Design review of the part built by this model. Coordinates are the model's own, in mm. Face numbers are marked on the shaded views. A direction names the side the tool comes from. Coordinates: 2 decimals unless noted, no trailing zeros. Loops run counter-clockwise (first coordinate to the right, second up) from the corner with the lowest first, then second, coordinate; pieces in that order, holes last. Notation, with made-up numbers: (39, 65.5) - (96, 65.5) arc R20 cw to (96, 83.5) - close; hole circle Ø4 at (31, -30). An arc over 180 degrees is marked (long way). Answer in a Markdown table with one row per item. Add a question column.
(1) We need section C-C, the plane y = -8.75. Write out the cut boundary in (x, z), plus the area to 3 significant figures.
(2) We need section D-D, the plane x = 28. Write out the cut boundary in (y, z), plus the area to 3 significant figures.
(3) We need section A-A, the plane y = -3.75. Write out the cut boundary in (x, z), plus the area to 3 significant figures.
(4) For the marked faces 1, 2 and 3, list the 3-axis set-ups (+Z, -Z, +X, -X, +Y, -Y) from which the entire face can be reached by the end or side of a thin tool; tool diameter is ignored.
(5) To check wall thickness, follow L1, parallel to X at y = -2.4, z = -89.63; L2, parallel to X at y = -7.8, z = -89.63; L3, parallel to Y at x = 27.5, z = -9. State the ranges of each line that lie inside material, in increasing order. Write a range as [from, to].
(6) We need section B-B, the plane z = -59.63. Write out the cut boundary in (x, y).
(7) Clearance check with flat-ended pins moving along their axes: pin 1 (2 mm diameter, centred on x = 28, y = -7, fed in from -Z); pin 2 (0.6 mm diameter, centred on x = 7, y = -10, fed in from -Z); pin 3 (7.5 mm diameter, centred on x = 5, z = -89.63, fed in from -Y); pin 4 (1.3 mm diameter, centred on x = 5.5, z = -39.5, fed in from -Y). State where each tip first meets the part, or that it passes through.
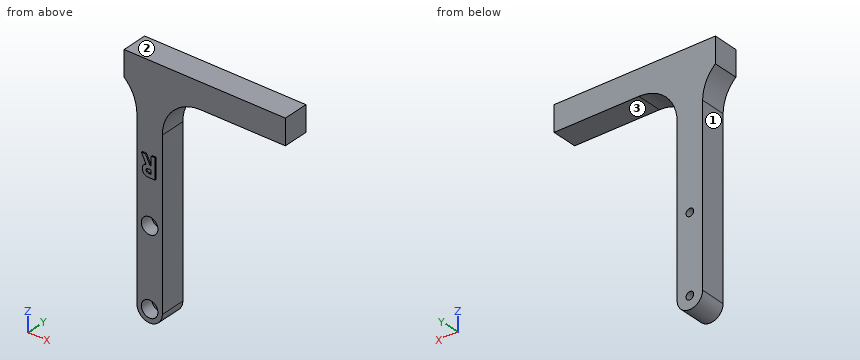
from build123d import *

# Parameters (mm, degrees)
BOSS_EXTRUDE1_DEPTH = 10
SKETCH2_R           = 1.5
CUT_EXTRUDE1_DEPTH  = 112.585820336
BOSS_EXTRUDE2_DEPTH = 0.5
SKETCH5_R           = 3.25
CUT_EXTRUDE2_DEPTH  = 5
FILLET1_R           = 15


with BuildPart() as part:
    # Sketch1 → Boss-Extrude1 (new body)
    with BuildSketch(Plane(origin=(0, 0, 0), x_dir=(1, 0, 0), z_dir=(0, 1, 0))):
        with BuildLine():
            Line((0, 0), (10, 0))
            Line((10, 0), (58.28, 0))
            Line((58.28, 0), (58.28, 10))
            Line((58.28, 10), (10, 10))
            Line((10, 10), (10, 89.63))
            ThreePointArc((10, 89.63), (5, 94.63), (0, 89.63))
            Line((0, 89.63), (0, 10))
            Line((0, 10), (-5, 10))
            Line((-5, 10), (-5, 0))
            Line((-5, 0), (0, 0))
        make_face()
    extrude(amount=BOSS_EXTRUDE1_DEPTH)

    # Sketch2 → Cut-Extrude1 (cut, through all)
    with BuildSketch(Plane(origin=(0, 10, 0), x_dir=(1, 0, 0), z_dir=(0, 1, 0))):
        with Locations(Location((5, 89.63, 0), (0, 0, 270))):
            Circle(SKETCH2_R)
        with Locations(Location((5, 59.63, 0), (0, 0, 270))):
            Circle(SKETCH2_R)
    extrude(amount=-CUT_EXTRUDE1_DEPTH, mode=Mode.SUBTRACT)

    # Sketch4 → Boss-Extrude2 (add)
    with BuildSketch(Plane(origin=(0, 10, 0), x_dir=(1, 0, 0), z_dir=(0, 1, 0))):
        with BuildLine():
            Line((7.461538462, 41.930004151), (5.788461538, 41.930004151))
            add(Edge.make_bspline(
                [(5.788461538, 41.930004151), (5.677871663, 41.92961162), (5.465176181, 41.928856674), (5.158480914, 41.916945611), (4.876739133, 41.900370391), (4.619533695, 41.875076164), (4.386974636, 41.841539077), (4.178828878, 41.802004401), (3.995102505, 41.756946162), (3.834246039, 41.700800041), (3.689081032, 41.637468067), (3.553767063, 41.564698468), (3.425318906, 41.483301557), (3.304595098, 41.391135559), (3.19054652, 41.289858519), (3.082958012, 41.179368492), (2.983349901, 41.058728567), (2.892338963, 40.928701036), (2.809389819, 40.791915054), (2.736080173, 40.648182815), (2.676464647, 40.497404362), (2.62378794, 40.341758769), (2.585846614, 40.179021052), (2.559458976, 40.010775491), (2.540138981, 39.836429843), (2.539028173, 39.71798715), (2.538461538, 39.657568254)],
                knots=[0, 0, 0, 0, 1.749336639, 3.364467119, 4.854658419, 6.213483162, 7.451590619, 8.570285859, 9.5643256, 10.440900261, 11.26203566, 12.067320669, 12.869050712, 13.665104639, 14.467235401, 15.27997916, 16.102287765, 16.939272006, 17.78853747, 18.631303466, 19.488103222, 20.351255419, 21.228522269, 22.127379805, 23.044756219, 24, 24, 24, 24], degree=3))
            add(Edge.make_bspline(
                [(2.538461538, 39.657568254), (2.539933452, 39.594504805), (2.542819606, 39.470848877), (2.558366003, 39.289208404), (2.586779932, 39.115427505), (2.629816962, 38.950014988), (2.679282438, 38.790912103), (2.745058832, 38.641054396), (2.819293994, 38.498262405), (2.907460927, 38.364555977), (3.004219829, 38.236965223), (3.116748396, 38.120378621), (3.237756507, 38.008530081), (3.374046466, 37.908425416), (3.519610488, 37.81329591), (3.677340774, 37.727083244), (3.846207924, 37.64762023), (3.964929894, 37.603306164), (4.025641026, 37.580645177)],
                knots=[0, 0, 0, 0, 1.099860209, 2.156625411, 3.176576793, 4.16617041, 5.135385252, 6.078461593, 7.016046972, 7.938469504, 8.868247731, 9.803980173, 10.76021508, 11.73834243, 12.748633912, 13.790971185, 14.870363756, 16, 16, 16, 16], degree=3))
            Line((4.025641026, 37.580645177), (2.179487179, 33.930004151))
            Line((2.179487179, 33.930004151), (3.775641026, 33.930004151))
            Line((3.775641026, 33.930004151), (5.538461538, 37.417183638))
            Line((5.538461538, 37.417183638), (6.025641026, 37.417183638))
            Line((6.025641026, 37.417183638), (6.025641026, 33.930004151))
            Line((6.025641026, 33.930004151), (7.461538462, 33.930004151))
            Line((7.461538462, 33.930004151), (7.461538462, 41.930004151))
        make_face()
        with BuildLine():
            Line((6.025641026, 38.853081074), (5.466346154, 38.853081074))
            add(Edge.make_bspline(
                [(5.466346154, 38.853081074), (5.397967707, 38.853851198), (5.267037673, 38.85532582), (5.078743088, 38.862165728), (4.907726699, 38.878646528), (4.753254104, 38.899469401), (4.61454801, 38.923512416), (4.492845628, 38.957967516), (4.386271709, 38.994887028), (4.296089158, 39.040768404), (4.219039259, 39.092945479), (4.152511603, 39.152219935), (4.097483692, 39.220822569), (4.052192915, 39.296889059), (4.016961614, 39.381092194), (3.991245464, 39.472507614), (3.976873938, 39.572176658), (3.975220446, 39.64096187), (3.974358974, 39.676799023)],
                knots=[0, 0, 0, 0, 1.688639943, 3.233382647, 4.650958383, 5.928841754, 7.082724185, 8.122798841, 9.049171256, 9.863274652, 10.613301712, 11.341792392, 12.054588806, 12.776240173, 13.521029143, 14.301969904, 15.115324896, 16, 16, 16, 16], degree=3))
            add(Edge.make_bspline(
                [(3.974358974, 39.676799023), (3.975987665, 39.719196991), (3.979186925, 39.802479943), (4.010933525, 39.922378191), (4.061467254, 40.033352223), (4.130735157, 40.134900631), (4.217969074, 40.223924975), (4.318076877, 40.302400643), (4.433219134, 40.36445333), (4.539832198, 40.405382621), (4.636825167, 40.429871039), (4.724358262, 40.448119591), (4.825722112, 40.461052863), (4.940993243, 40.474770901), (5.069877824, 40.483666354), (5.213078352, 40.490158262), (5.370183559, 40.49281442), (5.479700808, 40.493663547), (5.536858974, 40.494106715)],
                knots=[0, 0, 0, 0, 1.020303359, 2.004196876, 2.966617323, 3.9489082, 4.950758222, 5.960522915, 7.003732012, 8.091992268, 8.70421221, 9.413913587, 10.24622431, 11.166358409, 12.212345909, 13.359657661, 14.621978493, 16, 16, 16, 16], degree=3))
            Line((5.536858974, 40.494106715), (6.025641026, 40.494106715))
            Line((6.025641026, 40.494106715), (6.025641026, 38.853081074))
        make_face(mode=Mode.SUBTRACT)
    extrude(amount=BOSS_EXTRUDE2_DEPTH)

    # Sketch5 → Cut-Extrude2 (cut)
    with BuildSketch(Plane(origin=(0, 10, 0), x_dir=(1, 0, 0), z_dir=(0, 1, 0))):
        with Locations(Location((5, 89.63, 0), (0, 0, 270))):
            Circle(SKETCH5_R)
        with Locations(Location((5, 59.63, 0), (0, 0, 270))):
            Circle(SKETCH5_R)
    extrude(amount=-CUT_EXTRUDE2_DEPTH, mode=Mode.SUBTRACT)


with BuildPart() as body_2:
    # Mirror1: mirrored copy
    add(part.part.mirror(Plane.ZX))

    # Fillet1
    # the kernel refuses this fillet: 15 mm, written as the material it adds along each edge
    with BuildSketch(Plane(origin=(0, 0, -10), x_dir=(-1, 0, 0), z_dir=(0, -1, 0))) as fillet1_piece_1:
        with BuildLine():
            CenterArc((15, 11.180339887), FILLET1_R, 180, 48.189685104)
            Line((0, 11.180339887), (-0.3, 11.180339887))
            Line((-0.3, 11.180339887), (-0.3, 0))
            Line((-0.3, 0), (0, -0.3))
            ThreePointArc((0, -0.3), (2.5, -0.3), (4.8, -0.223606798))
            Line((4.8, -0.223606798), (5, 0))
        make_face()
    extrude(amount=10)
    with BuildSketch(Plane(origin=(10, 0, -10), x_dir=(1, 0, 0), z_dir=(0, -1, 0))) as fillet1_piece_2:
        with BuildLine():
            CenterArc((FILLET1_R, -FILLET1_R), FILLET1_R, 90, 90)
            Line((0, -FILLET1_R), (-FILLET1_R * 0.02, -FILLET1_R))
            Line((-FILLET1_R * 0.02, -FILLET1_R), (-FILLET1_R * 0.02, FILLET1_R * 0.02))
            Line((-FILLET1_R * 0.02, FILLET1_R * 0.02), (FILLET1_R, FILLET1_R * 0.02))
            Line((FILLET1_R, FILLET1_R * 0.02), (FILLET1_R, 0))
        make_face()
    extrude(amount=10)


solid = body_2.part
Responses:
| question | item | result |
|---|---|---|
| 1 | outline | (-5, -10) arc R15 cw to (0, -21.18) - (0, -89.63) arc R5 ccw to (10, -89.63) - (10, -25) arc R15 cw to (25, -10) - (58.28, -10) - (58.28, 0) - (-5, 0) - close; hole circle Ø6.5 at (5, -89.63); hole circle Ø6.5 at (5, -59.63) |
| 1 | area | 1,470 mm2 |
| 2 | outline | (-10, -10) - (0, -10) - (0, 0) - (-10, 0) - close |
| 2 | area | 100 mm2 |
| 3 | outline | (-5, -10) arc R15 cw to (0, -21.18) - (0, -89.63) arc R5 ccw to (10, -89.63) - (10, -25) arc R15 cw to (25, -10) - (58.28, -10) - (58.28, 0) - (-5, 0) - close; hole circle Ø3 at (5, -89.63); hole circle Ø3 at (5, -59.63) |
| 3 | area | 1,520 mm2 |
| 4 | face 1 | -Z, -X, +Y, -Y |
| 4 | face 2 | +Z, +X, -X, +Y, -Y |
| 4 | face 3 | -Z, +X, +Y, -Y |
| 5 | L1 | x = [0, 3.5], [6.5, 10] |
| 5 | L2 | x = [0, 1.75], [8.25, 10] |
| 5 | L3 | y = [-10, 0] |
| 6 | outline | (0, -10) - (1.75, -10) - (1.75, -5) - (3.5, -5) - (3.5, 0) - (0, 0) - close; (6.5, -5) - (8.25, -5) - (8.25, -10) - (10, -10) - (10, 0) - (6.5, 0) - close |
| 7 | pin 1 | stops at z = -10 |
| 7 | pin 2 | stops at z = -94.33 |
| 7 | pin 3 | stops at y = -10 |
| 7 | pin 4 | stops at y = -10.5 |
